Could you check a few things on this model? Use its own coordinates, in mm. A direction names the side the tool comes from. Coordinates: 2 decimals unless noted, no trailing zeros. Order: outer loops, then holes, each group sorted by start corner. A loop starts at its lowest first (then second) coordinate and runs counter-clockwise, first axis right, second up. Notation, with made-up numbers: (73.5, 62) -> (111.5, 62) arc R21 ccw to (111.5, 96) -> close; hole circle Ø2 at (-27, 6.5). An arc over 180 degrees is marked (long way). Put each result on its own line as item: value. Start each with the question number.
Q1. If we section it at D-D (x = 6): Please give me the cut outline in (y, z).
Q2. Will these pins go through, and if not, where does the flat tip stop? pin 1 (2.5 mm diameter, centred on y = -3, z = -21.5, fed in from +X); pin 2 (1.5 mm diameter, centred on y = -2, z = 61.5, fed in from -X); pin 3 (1.5 mm diameter, centred on x = 28, y = -3.5, fed in from -Z).
Q3. For faces 5 (the face through (13, -2, -30.053)), 6 (the face through (-21.284, -2.465, 32.339)), 7 (the face through (-15.242, -2, 62)), 8 (the face through (0, -2, -14.326)), 9 (the face through (-28, -2, -13.053)), which set-ups out of +Z, -Z, +X, -X, +Y, -Y let a thin tool reach every point of the face, with its end or its side?
Q4. If we section it at A-A (z = 51): Please give me the cut outline in (x, y), and give its area (3 significant figures).
Q5. If we section it at C-C (y = -3.3): Count the separate pieces of the cut face and the enclosed holes in it, and give its area (3 significant figures).
Q6. We'd pull the mould along Z, two halves only. Please class faces 1 (the face through (-13.257, -2.465, 24.463)), 2 (the face through (-10, -2, -35)), 3 (the face through (-21.497, -2.465, -28.914)), 4 (the face through (-16.916, -2.465, 12.13)): +Z half, -Z half, draft (parallel to the pull), parting line (faces both ways), or undercut.
Q7. If we section it at B-B (x = -26): Please give me the cut outline in (y, z), and give its area (3 significant figures).
Q8. Please list where these lines run through material, in increasing order: line 1 along Z through (x, y) = (13.5, -2.9); line 2 along Z through (x, y) = (0.5, -4.3); line 3 along X through (y, z) = (-0.9, 52).
from build123d import *

# Parameters (mm, degrees)
F1_DEPTH = 5


with BuildPart() as f1:
    # F0 (on Front) → F1 (new body)
    with BuildSketch(Plane.XZ):
        with BuildLine():
            ThreePointArc((-25, -25.864711), (-21.438301, -28.944777), (-16.861899, -30.053402))
            Line((-16.861899, -30.053402), (-10, -30.053402))
            Line((-10, -30.053402), (-10, -40.053402))
            Line((-10, -40.053402), (10, -40.053402))
            Line((10, -40.053402), (10, -30.053402))
            Line((10, -30.053402), (16.861899, -30.053402))
            ThreePointArc((16.861899, -30.053402), (21.438301, -28.944777), (25, -25.864711))
            Line((25, -25.864711), (25, -13.053402))
            Line((25, -13.053402), (30, -13.053402))
            Line((30, -13.053402), (30, 3.946598))
            Line((30, 3.946598), (23.767857, 3.946598))
            Line((23.767857, 3.946598), (18.868492, 59.946598))
            Line((18.868492, 59.946598), (25, 59.946598))
            Line((25, 59.946598), (27, 59.946598))
            Line((27, 59.946598), (25, 64.946598))
            Line((25, 64.946598), (21, 64.946598))
            Line((21, 64.946598), (15.242257, 64.946598))
            Line((15.242257, 64.946598), (15.242257, 59.946598))
            Line((15.242257, 59.946598), (18.308011, 24.904867))
            Line((18.308011, 24.904867), (8.346064, 24.03331))
            Line((8.346064, 24.03331), (10.448706, 0))
            Line((10.448706, 0), (10.524957, -0.871557))
            Line((10.524957, -0.871557), (20.486904, 0))
            Line((20.486904, 0), (21.373765, -10.136863))
            ThreePointArc((21.373765, -10.136863), (17.812066, -13.216929), (13.235664, -14.325554))
            Line((13.235664, -14.325554), (-13.235664, -14.325554))
            ThreePointArc((-13.235664, -14.325554), (-17.812066, -13.216929), (-21.373765, -10.136863))
            Line((-21.373765, -10.136863), (-20.486904, 0))
            Line((-20.486904, 0), (-10.524957, -0.871557))
            Line((-10.524957, -0.871557), (-10.448706, 0))
            Line((-10.448706, 0), (-8.346064, 24.03331))
            Line((-8.346064, 24.03331), (-18.308011, 24.904867))
            Line((-18.308011, 24.904867), (-15.242257, 59.946598))
            Line((-15.242257, 59.946598), (-15.242257, 64.946598))
            Line((-15.242257, 64.946598), (-21, 64.946598))
            Line((-21, 64.946598), (-25, 64.946598))
            Line((-25, 64.946598), (-27, 59.946598))
            Line((-27, 59.946598), (-25, 59.946598))
            Line((-25, 59.946598), (-18.868492, 59.946598))
            Line((-18.868492, 59.946598), (-23.767857, 3.946598))
            Line((-23.767857, 3.946598), (-30, 3.946598))
            Line((-30, 3.946598), (-30, -13.053402))
            Line((-30, -13.053402), (-25, -13.053402))
            Line((-25, -13.053402), (-25, -25.864711))
        make_face()
        Polygon((-17.560639, 4.763084), (-16.253303, 19.706005), (-11.272329, 19.270226), (-12.579665, 4.327305), align=None, mode=Mode.SUBTRACT)
        Polygon((16.253303, 19.706005), (17.560639, 4.763084), (12.579665, 4.327305), (11.272329, 19.270226), align=None, mode=Mode.SUBTRACT)
    extrude(amount=F1_DEPTH)


solid = f1.part
The answers:
1. outline: (-5, -40.05) -> (0, -40.05) -> (0, -14.33) -> (-5, -14.33) -> close
2. pin 1: x = 25
2. pin 2: x = -26.68
2. pin 3: z = -13.05
3. face 5: -Z, +X, +Y, -Y
3. face 6: -X, +Y, -Y
3. face 7: +Z, +Y, -Y
3. face 8: +Y, -Y
3. face 9: -Z, -X, +Y, -Y
4. outline: (-19.65, -5) -> (-16.02, -5) -> (-16.02, 0) -> (-19.65, 0) -> close; (16.02, -5) -> (19.65, -5) -> (19.65, 0) -> (16.02, 0) -> close
4. area: 36.3 mm^2
5. separate pieces: 1
5. enclosed holes: 2
5. area: 2,170 mm^2
6. face 1: undercut
6. face 2: draft
6. face 3: -Z half
6. face 4: undercut
7. outline: (-5, -13.05) -> (0, -13.05) -> (0, 3.95) -> (-5, 3.95) -> close; (-5, 59.95) -> (0, 59.95) -> (0, 62.45) -> (-5, 62.45) -> close
7. area: 97.5 mm^2
8. line 1: -30.05 to -14.32, -0.61 to 4.41, 19.47 to 24.48
8. line 2: -40.05 to -14.33
8. line 3: -19.56 to -15.94, 15.94 to 19.56
